from build123d import *

# Parameters (mm, degrees)
SKETCH1_W           = 140
SKETCH1_H           = 140
BOSS_EXTRUDE1_DEPTH = 140
SKETCH2_R           = 60
CUT_EXTRUDE1_DEPTH  = 130
CUT_EXTRUDE1_DRAFT  = -24
SKETCH3_R           = 10
BOSS_EXTRUDE2_DEPTH = 140
BOSS_EXTRUDE3_DEPTH = 140
SKETCH5_R           = 10
BOSS_EXTRUDE4_DEPTH = 40
FILLET1_R           = 30
FILLET2_R           = 1


with BuildPart() as part:
    # Sketch1 → Boss-Extrude1 (new body)
    with BuildSketch(Plane(origin=(0, 0, 0), x_dir=(0, 0, -1), z_dir=(1, 0, 0))):
        with Locations((70, -70)):
            Rectangle(SKETCH1_W, SKETCH1_H)
    extrude(amount=BOSS_EXTRUDE1_DEPTH)


with BuildPart() as cut_extrude1_tool:
    # Sketch2 → Cut-Extrude1 (with draft: the straight prism first)
    with BuildSketch(Plane.ZY):
        with Locations((-70, -70)):
            Circle(SKETCH2_R)
    extrude(amount=-CUT_EXTRUDE1_DEPTH)
    # Cut-Extrude1: the draft: its side faces are tilted about the plane it starts from
    cut_extrude1_sides = [cut_extrude1_tool.faces().sort_by_distance(p)[0] for p in [
        (65, -70, -130),
    ]]
    draft(cut_extrude1_sides, Plane.ZY, CUT_EXTRUDE1_DRAFT)


with BuildPart() as part_1:
    add(part.part)

    # Cut-Extrude1: cut by cut_extrude1_tool
    add(cut_extrude1_tool.part, mode=Mode.SUBTRACT)

    # Sketch3 → Boss-Extrude2 (add)
    with BuildSketch(Plane.XY):
        with Locations((20, -70)):
            Circle(SKETCH3_R)
    extrude(amount=-BOSS_EXTRUDE2_DEPTH)

    # Sketch4 → Boss-Extrude3 (add)
    with BuildSketch(Plane(origin=(0, -140, 0), x_dir=(-1, 0, 0), z_dir=(0, -1, 0))):
        with BuildLine():
            ThreePointArc((-210, 140), (-160.502525317, 119.497474683), (-140, 70))
            Line((-140, 70), (-140, 140))
            Line((-140, 140), (-210, 140))
        make_face()
        with BuildLine():
            Line((-210, 0), (-140, 0))
            Line((-140, 0), (-140, 70))
            ThreePointArc((-140, 70), (-160.502525317, 20.502525317), (-210, 0))
        make_face()
    extrude(amount=-BOSS_EXTRUDE3_DEPTH)

    # Sketch5 → Boss-Extrude4 (add)
    with BuildSketch(Plane(origin=(140, 0, 0), x_dir=(0, 0, -1), z_dir=(1, 0, 0))):
        with Locations(Location((70, -100, 0), (0, 0, 180))):
            Circle(SKETCH5_R)
        with Locations(Location((70, -40, 0), (0, 0, 180))):
            Circle(SKETCH5_R)
    extrude(amount=BOSS_EXTRUDE4_DEPTH)

    # Fillet1
    fillet1_edges = [part_1.edges().sort_by_distance(p)[0] for p in [
        (105, 0, -140),
        (105, -140, -140),
    ]]
    fillet(fillet1_edges, radius=FILLET1_R)

    # Fillet2
    fillet2_edges = [part_1.edges().sort_by_distance(p)[0] for p in [
        (0, -140, -55),
        (0, -70, 0),
        (0, 0, -55),
        (0, -70, -140),
        (0, -131.213203436, -131.213203436),
        (0, -8.786796564, -131.213203436),
        (105, 0, 0),
        (105, -140, 0),
    ]]
    fillet(fillet2_edges, radius=FILLET2_R)


solid = part_1.part
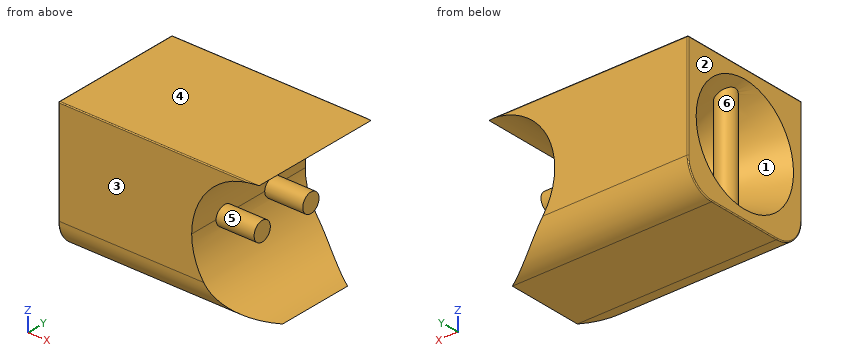
Verification items for the finished model (mm, model axes). Face numbers are marked on the shaded views. A direction names the side the tool comes from. Coordinates: 2 decimals unless noted, no trailing zeros. Write each loop counter-clockwise with the first axis right and the second up, starting at its lowest first coordinate (ties: lowest second). Pieces come first, ordered by that corner, then holes. Notation, with made-up numbers: (54.25, 11.5) - (111.25, 11.5) arc R27 cw to (111.25, 50.5) - close; hole circle Ø9 at (11, 68). An arc over 180 degrees is marked (long way). Answer as a JSON object with one key per item and string values.
(1) Tool access check on the marked faces 4, 5 and 6. Record the directions out of +Z, -Z, +X, -X, +Y, -Y that give a thin tool (end or side, any length) a straight path to the whole face; none if there is none.
Report:
{"face 4": "+Z, +X, -X, +Y, -Y", "face 5": "+X", "face 6": "none"}
(2) Cross-section at A-A on x = 54. Record the cut outline in (y, z), plus the area to 3 significant figures.
Report:
{"outline": "(-140, -110) arc R30 ccw to (-110, -140) - (-30, -140) arc R30 ccw to (0, -110) - (0, -1) arc R1 ccw to (-1, 0) - (-139, 0) arc R1 ccw to (-140, -1) - close; hole circle Ø71.92 at (-70, -70)", "area": "15,200 mm^2"}
(3) Gauge pin test, flat ends, axial feed: pin 1 Ø6 at (x, z) = (159.5, -27.5) entering from +Y; pin 2 Ø8 at (y, z) = (-41, -79) entering from +X; pin 3 Ø3 at (y, z) = (-22.5, -55.5) entering from +X; pin 4 Ø1.5 at (y, z) = (-20, -29) entering from +X. Record the tip position at first contact, or that the pin passes through.
Report:
{"pin 1": "through", "pin 2": "x = 180", "pin 3": "x = 141.85", "pin 4": "x = 153.81"}
(4) Thickness scan on line 1 along Z through (x, y) = (154, -102.5); line 2 along Z through (x, y) = (88.5, -77); line 3 along X through (y, z) = (-68, -72.5). Record the ranges inside material, lowest first.
Report:
{"line 1": "-140 to -112, -79.68 to -60.32, -28 to 0", "line 2": "-140 to -89.37, -50.63 to 0", "line 3": "10.2 to 29.8, 127.57 to 140.04"}
(5) Cross-section at C-C on x = 17.5. Record the cut outline in (y, z), plus the area to 3 significant figures.
Report:
{"outline": "(-140, -110) arc R30 ccw to (-110, -140) - (-30, -140) arc R30 ccw to (0, -110) - (0, -1) arc R1 ccw to (-1, 0) - (-139, 0) arc R1 ccw to (-140, -1) - close; hole (-79.68, -121.3) - (-79.68, -18.7) arc R52.21 ccw to start; hole (-60.32, -121.3) arc R52.21 ccw to (-60.32, -18.7) - close", "area": "12,700 mm^2"}
(6) Cross-section at B-B on x = 188. Record the cut outline in (y, z).
Report:
{"outline": "(-140, -3.55) - (0, -3.55) - (0, -1) arc R1 ccw to (-1, 0) - (-139, 0) arc R1 ccw to (-140, -1) - close; (-124.15, -136.45) arc R30 ccw to (-110, -140) - (-30, -140) arc R30 ccw to (-15.85, -136.45) - close"}
(7) Cross-section at D-D on x = 98.5. Record the cut outline in (y, z), plus the area to 3 significant figures.
Report:
{"outline": "(-140, -110) arc R30 ccw to (-110, -140) - (-30, -140) arc R30 ccw to (0, -110) - (0, -1) arc R1 ccw to (-1, 0) - (-139, 0) arc R1 ccw to (-140, -1) - close; hole circle Ø32.29 at (-70, -70)", "area": "18,400 mm^2"}
(8) Mould release check, pull along Y, two halves, no side actions. Record for the marked faces 1, 2 and 3: pulls with the +Y half, pulls with the -Y half, needs draft (parallel to the pull), parting line crosses it, or undercut.
Report:
{"face 1": "undercut", "face 2": "needs draft", "face 3": "pulls with the -Y half"}
